```python
from build123d import *

# Parameters (mm, degrees)
F0_W     = 101.6
F0_H     = 76.2
F1_DEPTH = 63.5
F3_DEPTH = 101.6
F4_W     = 50.8
F4_H     = 25.4
F5_DEPTH = 38.1


with BuildPart() as f1:
    # F0 (on Front) → F1 (new body)
    with BuildSketch(Plane.XZ):
        with Locations((-2.540003, -7.110645)):
            Rectangle(F0_W, F0_H)
    extrude(amount=F1_DEPTH)

    # F2 (on face) → F3 (cut)
    with BuildSketch(Plane(origin=(-53.340003, 0, 0), x_dir=(0, -1, 0), z_dir=(-1, 0, 0))):
        with BuildLine():
            Line((63.5, 30.989355), (12.7, 30.989355))
            ThreePointArc((12.7, 30.989355), (27.666821, -4.843824), (63.5, -19.810645))
            Line((63.5, -19.810645), (63.5, 30.989355))
        make_face()
    extrude(amount=-F3_DEPTH, mode=Mode.SUBTRACT)

    # F4 (on face) → F5 (cut)
    with BuildSketch(Plane.XY.offset(30.989355)):
        with Locations((-2.540003, -12.7)):
            Rectangle(F4_W, F4_H)
    extrude(amount=-F5_DEPTH, mode=Mode.SUBTRACT)


solid = f1.part
```
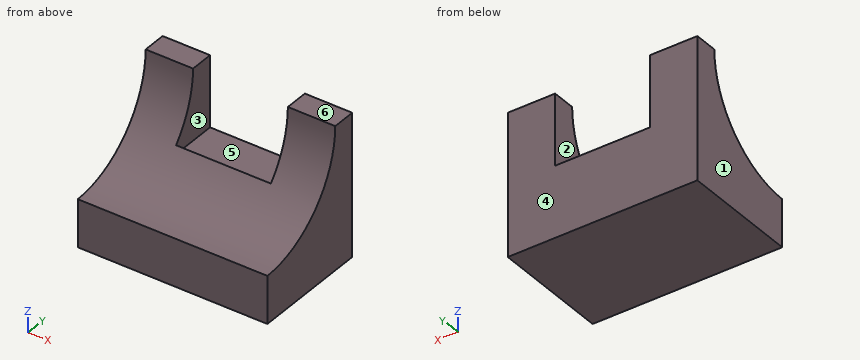
Model file for the job. Use its own axes, mm. Face numbers are marked on the shaded views. A direction names the side the tool comes from. Round coordinates to 2 decimals unless told otherwise and drop trailing zeros. Order: outer loops, then holes, each group sorted by start corner. A loop starts at its lowest first (then second) coordinate and runs counter-clockwise, first axis right, second up. Notation, with made-up numbers: M 11,43 L 65,43 A27 cw 65,60 Z; hole C -11,4.25 d2. An arc over 180 degrees is marked long. Use CSV: the item, a comma, the result in double quotes.
Item 1: Probe probe 1 along X at (y, z) = (-18, -5.5); probe 2 along Z at (x, y) = (-9, -14.5); probe 3 along Z at (x, y) = (34, -40). List the from-to ranges inside material, lowest first.
Worked answers:
probe 1,"-53.34 to -27.94, 22.86 to 48.26"
probe 2,"-45.21 to -7.11"
probe 3,"-45.21 to -13.93"
Item 2: Pull direction X, two halves, no side cores. Call the marked faces 1, 2, 3 and 4: released by +X, released by -X, zero draft, split by the parting line, or undercut.
Worked answers:
face 1,"released by -X"
face 2,"undercut"
face 3,"undercut"
face 4,"zero draft"
Item 3: Pin check, flat tips, straight feed: pin 1 (3 mm diameter, centred on x = -7.5, z = -0.5, fed in from -Y); pin 2 (8 mm diameter, centred on x = -5, z = -11, fed in from -Y). Stop position of each tip, or through.
Worked answers:
pin 1,"through"
pin 2,"y = -42.15"
Item 4: Saw through at A-A (z = 25.5). List the corners of the cut face in (x, y), plus the area to 3 significant figures.
Worked answers:
outline,"M -53.34,-13.03 L -27.94,-13.03 L -27.94,0 L -53.34,0 Z; M 22.86,-13.03 L 48.26,-13.03 L 48.26,0 L 22.86,0 Z"
area,"662 mm²"
Item 5: Saw through at B-B (x = 36.5). List the corners of the cut face in (y, z).
Worked answers:
outline,"M -63.5,-45.21 L 0,-45.21 L 0,30.99 L -12.7,30.99 A51.1 cw -63.5,-19.81 Z"
Item 6: Saw through at D-D (y = -30.5). List the corners of the cut face in (x, z), plus the area to 3 significant figures.
Worked answers:
outline,"M -53.34,-45.21 L 48.26,-45.21 L 48.26,-7.47 L -53.34,-7.47 Z"
area,"3,830 mm²"
Item 7: Saw through at C-C (z = 9). List the corners of the cut face in (x, y).
Worked answers:
outline,"M -53.34,-17.82 L -27.94,-17.82 L -27.94,0 L -53.34,0 Z; M 22.86,-17.82 L 48.26,-17.82 L 48.26,0 L 22.86,0 Z"
Item 8: Which spindle directions (+Z, -Z, +X, -X, +Y, -Y) get a long thin tool onto all of the face, cutting with end or side? Do the marked faces 5 and 6. Say none if no direction does.
Worked answers:
face 5,"+Z, +Y"
face 6,"+Z, +X, -X, +Y, -Y"
